Geometry: final body of the model. Coordinates: model frame, mm. A direction names the side the tool comes from. Give positions to 0.01 mm unless a question says otherwise; leave off trailing zeros. Write each loop counter-clockwise with the first axis right and the second up, starting at its lowest first coordinate (ties: lowest second). Pieces come first, ordered by that corner, then holes. Notation, with made-up numbers: M 69.5,85.25 L 126.5,85.25 A17 ccw 126.5,106.25 Z; hole C -21,2.5 d5. An arc over 180 degrees is marked long. Use a Markdown table: item, result. Add a question column.
1) Section D-D on y = 20.5. Return the cut outline in (x, z), then the cut area to 3 significant figures.
2) Section A-A on z = 0. Return the cut outline in (x, y), then the cut area to 3 significant figures.
3) Section C-C on x = 0. Return the cut outline in (y, z), then the cut area to 3 significant figures.
4) Section B-B on y = 17.5. Return the cut outline in (x, z).
5) Pin query (flat end, axial travel): pin 1 (3.5 mm diameter, centred on y = 20, z = 0, fed in from +X); pin 2 (3 mm diameter, centred on x = 6.5, z = 8, fed in from -Y); pin 3 (3 mm diameter, centred on x = 7.5, y = 19, fed in from -Z); pin 4 (3 mm diameter, centred on x = 6.5, y = 20.5, fed in from +Z). Return the tip coordinate at first contact, or that it passes through.
6) Set-up query: faces 1 (the cylindrical face through (7.535, 15.141, 7.703)), 2 (the cylindrical face through (1.397, 5.916, 4.435)), 3 (the flat face through (7, 20, -6.5)). Return all of +Z, -Z, +X, -X, +Y, -Y with unobstructed straight access to the full face (end or side cutting, diameter ignored); none if empty.
7) Draft query along Y for faces 4 (the cylindrical face through (7.535, 24.797, -5.359)), 5 (the cylindrical face through (7.5, 21.4, 1.5)), 6 (the flat face through (10, 17.5, -0.2)), 7 (the flat face through (5, 12, -4)). Return one class per face: +Y half, -Y half, draft (parallel to the pull), parting line (faces both ways), or undercut.
8) Line query: line 1 (X direction, y = 20, z = -3.5); line 2 (Y direction, x = -6.5, z = -13.5); line 3 (Y direction, x = 2.75, z = 1.5). Output: solid intervals per line, ascending.
```python
from build123d import *

# Parameters (mm, degrees)
SKETCH1_R           = 4.65
BOSS_EXTRUDE1_DEPTH = 12
SKETCH2_R           = 17.5
BOSS_EXTRUDE2_DEPTH = 2
SKETCH3_W           = 5
SKETCH3_H           = 13
BOSS_EXTRUDE3_DEPTH = 12
FILLET1_R           = 4
FILLET2_R           = 4
CUT_EXTRUDE1_DEPTH  = 29.434134416
SKETCH5_R           = 2.05
CUT_EXTRUDE2_DEPTH  = 70
FILLET3_R           = 4


with BuildPart() as part:
    # Sketch1 → Boss-Extrude1 (new body)
    with BuildSketch(Plane(origin=(0, 0, 0), x_dir=(1, 0, 0), z_dir=(0, 1, 0))):
        with Locations(Location((0, 0, 0), (0, 0, 270))):
            Circle(SKETCH1_R)
    extrude(amount=BOSS_EXTRUDE1_DEPTH)

    # Sketch2 → Boss-Extrude2 (add)
    with BuildSketch(Plane(origin=(0, 12, 0), x_dir=(1, 0, 0), z_dir=(0, 1, 0))):
        with Locations(Location((0, 0, 0), (0, 0, 270))):
            Circle(SKETCH2_R)
    extrude(amount=BOSS_EXTRUDE2_DEPTH)

    # Sketch3 → Boss-Extrude3 (add)
    with BuildSketch(Plane(origin=(0, 14, 0), x_dir=(1, 0, 0), z_dir=(0, 1, 0))):
        with Locations((7.5, 0)):
            Rectangle(SKETCH3_W, SKETCH3_H)
    boss_extrude3 = extrude(amount=BOSS_EXTRUDE3_DEPTH)

    # Mirror1: Boss-Extrude3 across plane
    add(boss_extrude3.mirror(Plane(origin=(0, 0, 0), x_dir=(0, 0, 1), z_dir=(1, 0, 0))))

    # Fillet1
    fillet1_edges = [part.edges().sort_by_distance(p)[0] for p in [
        (7.5, 26, -6.5),
        (7.5, 26, 6.5),
        (-7.5, 26, 6.5),
        (-7.5, 26, -6.5),
    ]]
    fillet(fillet1_edges, radius=FILLET1_R)

    # Fillet2
    fillet2_edges = [part.edges().sort_by_distance(p)[0] for p in [
        (7.5, 14, 6.5),
        (7.5, 14, -6.5),
        (-7.5, 14, -6.5),
        (-7.5, 14, 6.5),
    ]]
    fillet(fillet2_edges, radius=FILLET2_R)

    # Sketch4 → Cut-Extrude1 (cut, through all)
    with BuildSketch(Plane(origin=(0, 14, 0), x_dir=(1, 0, 0), z_dir=(0, 1, 0))):
        with BuildLine():
            Line((10, 14.361406616), (10, 0))
            Line((10, 0), (10, -14.361406616))
            ThreePointArc((10, -14.361406616), (15.512092057, -8.100925873), (17.5, 0))
            ThreePointArc((17.5, 0), (15.512092057, 8.100925873), (10, 14.361406616))
        make_face()
    cut_extrude1 = extrude(amount=-CUT_EXTRUDE1_DEPTH, mode=Mode.SUBTRACT)

    # Mirror2: Cut-Extrude1 across plane
    add(cut_extrude1.mirror(Plane(origin=(0, 0, 0), x_dir=(0, 0, 1), z_dir=(1, 0, 0))), mode=Mode.SUBTRACT)

    # Sketch5 → Cut-Extrude2 (cut)
    with BuildSketch(Plane(origin=(10, 0, 0), x_dir=(0, 0, -1), z_dir=(1, 0, 0))):
        with Locations((0, 20)):
            Circle(SKETCH5_R)
    extrude(amount=-CUT_EXTRUDE2_DEPTH, mode=Mode.SUBTRACT)

    # Fillet3
    fillet3_edges = [part.edges().sort_by_distance(p)[0] for p in [
        (10, 13, -14.361406616),
        (10, 13, 14.361406616),
        (-10, 13, 14.361406616),
        (-10, 13, -14.361406616),
    ]]
    fillet(fillet3_edges, radius=FILLET3_R)


solid = part.part
```
Found:
| question | item | result |
|---|---|---|
| 1 | outline | M -10,-6.5 L -5,-6.5 L -5,-1.99 L -10,-1.99 Z; M -10,1.99 L -5,1.99 L -5,6.5 L -10,6.5 Z; M 5,-6.5 L 10,-6.5 L 10,-1.99 L 5,-1.99 Z; M 5,1.99 L 10,1.99 L 10,6.5 L 5,6.5 Z |
| 1 | area | 90.2 mm² |
| 2 | outline | M -10,12 L -4.65,12 L -4.65,0 L 4.65,0 L 4.65,12 L 10,12 L 10,17.95 L 5,17.95 L 5,14 L -5,14 L -5,17.95 L -10,17.95 Z; M -10,22.05 L -5,22.05 L -5,26 L -10,26 Z; M 5,22.05 L 10,22.05 L 10,26 L 5,26 Z |
| 2 | area | 231 mm² |
| 3 | outline | M 0,-4.65 L 12,-4.65 L 12,-17.5 L 14,-17.5 L 14,17.5 L 12,17.5 L 12,4.65 L 0,4.65 Z |
| 3 | area | 182 mm² |
| 4 | outline | M -10,-6.53 L -5,-6.53 L -5,6.53 L -10,6.53 Z; M 5,-6.53 L 10,-6.53 L 10,6.53 L 5,6.53 Z |
| 5 | pin 1 | through |
| 5 | pin 2 | y = 12 |
| 5 | pin 3 | z = -6.53 |
| 5 | pin 4 | z = 6.5 |
| 6 | face 1 | +Z, +X, -X, +Y |
| 6 | face 2 | -Y |
| 6 | face 3 | -Z, +X, -X, +Y |
| 7 | face 4 | +Y half |
| 7 | face 5 | undercut |
| 7 | face 6 | draft |
| 7 | face 7 | -Y half |
| 8 | line 1 | -10 to -5, 5 to 10 |
| 8 | line 2 | 12 to 14 |
| 8 | line 3 | 0 to 14 |
